```python
from build123d import *

# Parameters (mm, degrees)
F0_W     = 457.2
F0_H     = 457.2
F1_DEPTH = 6.35
F3_DEPTH = 15.875
F5_DEPTH = 15.875
F7_DEPTH = 15.875


with BuildPart() as f1:
    # F0 (on Top) → F1 (new body)
    with BuildSketch(Plane.XY):
        Rectangle(F0_W, F0_H)
    extrude(amount=F1_DEPTH)

    # F2 (on face) → F3 (join)
    with BuildSketch(Plane.XY.offset(6.35)):
        Polygon((76.373018, 5.326067), (102.837036, -144.758628), (202.893499, -127.11595), (176.429482, 22.968745), align=None)
    extrude(amount=F3_DEPTH)

    # F4 (on face) → F5 (join)
    with BuildSketch(Plane.XY.offset(6.35)):
        Polygon((228.6, -122.583194), (202.893499, -127.11595), (102.837036, -144.758628), (-228.6, -203.2), (-228.6, -228.6), (228.6, -228.6), align=None)
    extrude(amount=F5_DEPTH)

    # F6 (on face) → F7 (join)
    with BuildSketch(Plane.XY.offset(6.35)):
        Polygon((-228.6, -203.2), (102.837036, -144.758628), (76.373018, 5.326067), (42.190329, 199.185465), (-228.6, 151.437759), align=None)
    extrude(amount=F7_DEPTH)


solid = f1.part
```
Can you work these out from the model? Positions are in its coordinate system, mm. A direction names the side the tool comes from. Coordinates: 2 decimals unless noted, no trailing zeros. Order: outer loops, then holes, each group sorted by start corner. A loop starts at its lowest first (then second) coordinate and runs counter-clockwise, first axis right, second up.
1. Thinking about a two-plate mould opening in X: for faces 4 (the face through (127.1, 14.27, 14.18)), 5 (the face through (-3, -228.6, 11)), 6 (the face through (228.6, -54, 6)), 7 (the face through (215.927, -124.818, 14.176)), which applies, +X half, -X half, draft (parallel to the pull), parting line (faces both ways), or undercut?
2. If we section it at C-C (y = 143.5): Please give me the cut outline in (x, z) (3 decimals).
3. For faces 1 (the face through (84, 131, 6.35)), 2 (the face through (-91.309, 175.646, 14.176)), 3 (the face through (-54, -59, 22.225)), which set-ups out of +Z, -Z, +X, -X, +Y, -Y let a thin tool reach every point of the face, with its end or its side?
4. If we section it at A-A (z = 10.25): Please give me the cut outline in (x, y).
5. I need wall thicknesses on line 1 (Z direction, x = 178, y = 117); line 2 (Y direction, x = 157, z = 21.25). Which ranges of each line are inside material? Lowest first, please.
6. If we section it at B-B (x = -40.5): Please give me the cut outline in (y, z) (3 decimals).
7. I'm going to push a flat-ended pin straight in: pin 1 (2 mm diameter, centred on y = -73, z = 13, fed in from +X). Where does the tip first touch, or does it pass through?
Entries:
1. face 4: undercut
1. face 5: draft
1. face 6: +X half
1. face 7: undercut
2. outline: (-228.6, 0) - (228.6, 0) - (228.6, 6.35) - (52.009, 6.35) - (52.009, 22.225) - (-228.6, 22.225) - close
3. face 1: +Z, +Y
3. face 2: +Z, -X, +Y
3. face 3: +Z, +X, -X, +Y, -Y
4. outline: (-228.6, -228.6) - (228.6, -228.6) - (228.6, -122.58) - (202.89, -127.12) - (176.43, 22.97) - (76.37, 5.33) - (42.19, 199.19) - (-228.6, 151.44) - close
5. line 1: z = 0 to 6.35
5. line 2: y = -228.6 to 19.54
6. outline: (-228.6, 0) - (228.6, 0) - (228.6, 6.35) - (184.605, 6.35) - (184.605, 22.225) - (-228.6, 22.225) - close
7. pin 1: stops at x = 193.53
